Model file for the job. Use its own axes, mm. A direction names the side the tool comes from. Coordinates: 2 decimals unless noted, no trailing zeros. Loops run counter-clockwise (first coordinate to the right, second up) from the corner with the lowest first, then second, coordinate; pieces in that order, holes last. Notation, with made-up numbers: M 54.5,65.5 L 92.5,65.5 A25 ccw 92.5,86.5 Z; hole C 53,-20.75 d11. An arc over 180 degrees is marked long. Write item = value, one per line. Start each with the question number.
from build123d import *

# Parameters (mm, degrees)
F0_R     = 5
F1_DEPTH = 6.75
F0_R_2   = 4.5
F2_DEPTH = 2.75
F3_R     = 5.154476
F4_DEPTH = 13.501


with BuildPart() as f1:
    # F0 (on Top) → F1 (new body, symmetric)
    with BuildSketch(Plane.XY):
        with BuildLine():
            Line((-21.880162, -1), (-18.007179, -2))
            ThreePointArc((-18.007179, -2), (-17.769775, -3.534628), (-17.401831, -5.04329))
            Line((-17.401831, -5.04329), (-20.597318, -7.449296))
            Line((-20.597318, -7.449296), (-19.831951, -9.297055))
            Line((-19.831951, -9.297055), (-15.871097, -8.738808))
            ThreePointArc((-15.871097, -8.738808), (-15.064488, -10.065769), (-14.147212, -11.318785))
            Line((-14.147212, -11.318785), (-16.178718, -14.764504))
            Line((-16.178718, -14.764504), (-14.764504, -16.178718))
            Line((-14.764504, -16.178718), (-11.318785, -14.147212))
            ThreePointArc((-11.318785, -14.147212), (-10.065769, -15.064488), (-8.738808, -15.871097))
            Line((-8.738808, -15.871097), (-9.297055, -19.831951))
            Line((-9.297055, -19.831951), (-7.449296, -20.597318))
            Line((-7.449296, -20.597318), (-5.04329, -17.401831))
            ThreePointArc((-5.04329, -17.401831), (-3.534628, -17.769775), (-2, -18.007179))
            Line((-2, -18.007179), (-1, -21.880162))
            Line((-1, -21.880162), (1, -21.880162))
            Line((1, -21.880162), (2, -18.007179))
            ThreePointArc((2, -18.007179), (3.534628, -17.769775), (5.04329, -17.401831))
            Line((5.04329, -17.401831), (7.449296, -20.597318))
            Line((7.449296, -20.597318), (9.297055, -19.831951))
            Line((9.297055, -19.831951), (8.738808, -15.871097))
            ThreePointArc((8.738808, -15.871097), (10.065769, -15.064488), (11.318785, -14.147212))
            Line((11.318785, -14.147212), (14.764504, -16.178718))
            Line((14.764504, -16.178718), (16.178718, -14.764504))
            Line((16.178718, -14.764504), (14.147212, -11.318785))
            ThreePointArc((14.147212, -11.318785), (15.064488, -10.065769), (15.871097, -8.738808))
            Line((15.871097, -8.738808), (19.831951, -9.297055))
            Line((19.831951, -9.297055), (20.597318, -7.449296))
            Line((20.597318, -7.449296), (17.401831, -5.04329))
            ThreePointArc((17.401831, -5.04329), (17.769775, -3.534628), (18.007179, -2))
            Line((18.007179, -2), (21.880162, -1))
            Line((21.880162, -1), (21.880162, 1))
            Line((21.880162, 1), (18.007179, 2))
            ThreePointArc((18.007179, 2), (17.769775, 3.534628), (17.401831, 5.04329))
            Line((17.401831, 5.04329), (20.597318, 7.449296))
            Line((20.597318, 7.449296), (19.831951, 9.297055))
            Line((19.831951, 9.297055), (15.871097, 8.738808))
            ThreePointArc((15.871097, 8.738808), (15.064488, 10.065769), (14.147212, 11.318785))
            Line((14.147212, 11.318785), (16.178718, 14.764504))
            Line((16.178718, 14.764504), (14.764504, 16.178718))
            Line((14.764504, 16.178718), (11.318785, 14.147212))
            ThreePointArc((11.318785, 14.147212), (10.065769, 15.064488), (8.738808, 15.871097))
            Line((8.738808, 15.871097), (9.297055, 19.831951))
            Line((9.297055, 19.831951), (7.449296, 20.597318))
            Line((7.449296, 20.597318), (5.04329, 17.401831))
            ThreePointArc((5.04329, 17.401831), (3.534628, 17.769775), (2, 18.007179))
            Line((2, 18.007179), (1, 21.880162))
            Line((1, 21.880162), (-1, 21.880162))
            Line((-1, 21.880162), (-2, 18.007179))
            ThreePointArc((-2, 18.007179), (-3.534628, 17.769775), (-5.04329, 17.401831))
            Line((-5.04329, 17.401831), (-7.449296, 20.597318))
            Line((-7.449296, 20.597318), (-9.297055, 19.831951))
            Line((-9.297055, 19.831951), (-8.738808, 15.871097))
            ThreePointArc((-8.738808, 15.871097), (-10.065769, 15.064488), (-11.318785, 14.147212))
            Line((-11.318785, 14.147212), (-14.764504, 16.178718))
            Line((-14.764504, 16.178718), (-16.178718, 14.764504))
            Line((-16.178718, 14.764504), (-14.147212, 11.318785))
            ThreePointArc((-14.147212, 11.318785), (-15.064488, 10.065769), (-15.871097, 8.738808))
            Line((-15.871097, 8.738808), (-19.831951, 9.297055))
            Line((-19.831951, 9.297055), (-20.597318, 7.449296))
            Line((-20.597318, 7.449296), (-17.401831, 5.04329))
            ThreePointArc((-17.401831, 5.04329), (-17.769775, 3.534628), (-18.007179, 2))
            Line((-18.007179, 2), (-21.880162, 1))
            Line((-21.880162, 1), (-21.880162, -1))
        make_face()
        Circle(F0_R, mode=Mode.SUBTRACT)
    extrude(amount=F1_DEPTH, both=True)

    # F0 (on Top) → F2 (join, symmetric)
    with BuildSketch(Plane.XY):
        Circle(F0_R)
        Circle(F0_R_2, mode=Mode.SUBTRACT)
    extrude(amount=F2_DEPTH, both=True)

    # F3 (on face) → F4 (cut, through all)
    with BuildSketch(Plane.XY.offset(6.75)):
        with Locations((0, 11.558953)):
            Circle(F3_R)
        with Locations((-10.010347, 5.779476)):
            Circle(F3_R)
        with Locations((-10.010347, -5.779476)):
            Circle(F3_R)
        with Locations((0, -11.558953)):
            Circle(F3_R)
        with Locations((10.010347, -5.779476)):
            Circle(F3_R)
        with Locations((10.010347, 5.779476)):
            Circle(F3_R)
    extrude(amount=-F4_DEPTH, mode=Mode.SUBTRACT)


solid = f1.part
Item 1: Cut at D-D (z = -5.5). Give the number of separate pieces and of enclosed holes in the cut face, plus the area to 3 significant figures.
Item 2: Probe L1, parallel to Y at x = 0, z = 4.85; L2, parallel to Y at x = 0, z = -1.5; L3, parallel to X at y = 6, z = 1. List the from-to ranges inside material, lowest first.
Item 3: Cut at C-C (y = -13). Give the cut face in (x, z), plus the area to 3 significant figures.
Item 4: Pull direction X, two halves, no side cores. Call faces 1 (the flat face through (17.88, 9.02, 0.09)), 2 (the flat face through (-15.15, -13.02, 0.09)), 3 (the flat face through (8.36, -20.22, 0.09)): +X half, -X half, draft (parallel to the pull), parting line (faces both ways), or undercut.
Item 5: 3-axis set-ups, long thin cutter, end or side, ignore diameter. For faces 4 (the cylindrical face through (-1.08, -4.88, -4.78)), 5 (the flat face through (15.15, 13.02, 0.09)), 6 (the flat face through (-1.507, -19.917, 0.095)), 7 (the flat face through (-19.971, -1.493, 0.095)): which of +Z, -Z, +X, -X, +Y, -Y reach the whole face in a straight line?
Item 6: Pin check, flat tips, straight feed: pin 1 Ø8 at (x, y) = (-10.01, 5.78) entering from +Z; pin 2 Ø8 at (y, z) = (-7.5, 4) entering from -X; pin 3 Ø4 at (y, z) = (10.5, 1) entering from +X; pin 4 Ø2 at (x, z) = (17, 5) entering from -Y. Stop position of each tip, or through.
Item 7: Cut at B-B (y = 0). Give the cut face in (x, z).
Item 8: Cut at A-A (x = 0). Give the cut face in (y, z), plus the area to 3 significant figures.
Reported:
q1.separate_pieces = 1
q1.enclosed_holes = 7
q1.area = 633 mm^2
q2.L1 = -21.88 to -16.71, -6.4 to -5, 5 to 6.4, 16.71 to 21.88
q2.L2 = -21.88 to -16.71, -6.4 to -4.5, 4.5 to 6.4, 16.71 to 21.88
q2.L3 = -18.67 to -15.16, -4.86 to 4.86, 15.16 to 18.67
q3.outline = M -15.14,-6.75 L -4.95,-6.75 L -4.95,6.75 L -15.14,6.75 Z; M 4.95,-6.75 L 15.14,-6.75 L 15.14,6.75 L 4.95,6.75 Z
q3.area = 275 mm^2
q4.face_1 = undercut
q4.face_2 = -X half
q4.face_3 = +X half
q5.face_4 = -Z
q5.face_5 = +Z, -Z, +X
q5.face_6 = +Z, -Z, -Y
q5.face_7 = +Z, -Z, -X
q6.pin_1 = through
q6.pin_2 = -20.6
q6.pin_3 = 20.16
q6.pin_4 = -14.94
q7.outline = M -21.88,-6.75 L -5,-6.75 L -5,-2.75 L -4.5,-2.75 L -4.5,2.75 L -5,2.75 L -5,6.75 L -21.88,6.75 Z; M 4.5,-2.75 L 5,-2.75 L 5,-6.75 L 21.88,-6.75 L 21.88,6.75 L 5,6.75 L 5,2.75 L 4.5,2.75 Z
q8.outline = M -21.88,-6.75 L -16.71,-6.75 L -16.71,6.75 L -21.88,6.75 Z; M -6.4,-6.75 L -5,-6.75 L -5,-2.75 L -4.5,-2.75 L -4.5,2.75 L -5,2.75 L -5,6.75 L -6.4,6.75 Z; M 4.5,-2.75 L 5,-2.75 L 5,-6.75 L 6.4,-6.75 L 6.4,6.75 L 5,6.75 L 5,2.75 L 4.5,2.75 Z; M 16.71,-6.75 L 21.88,-6.75 L 21.88,6.75 L 16.71,6.75 Z
q8.area = 183 mm^2
